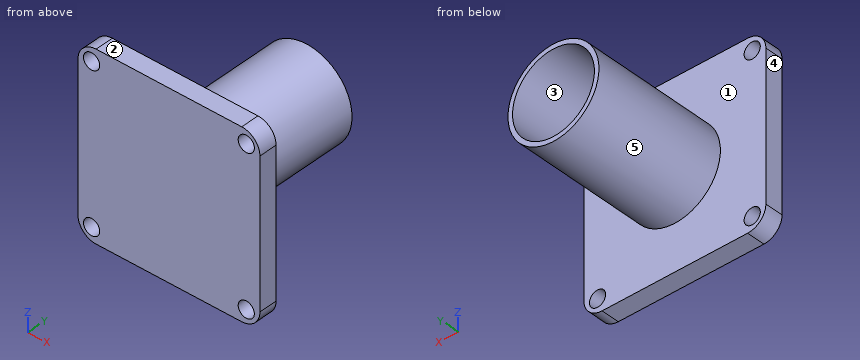
Autodesk Inventor part; units mm, degrees
ref_plane "YZ Plane" through (0, 0, 0) normal (1, 0, 0) x (0, 1, 0)
ref_plane "XZ Plane" through (0, 0, 0) normal (0, 1, 0) x (-1, 0, 0)
sketch "Sketch1" plane through (0, 0, 0) normal (0, 1, 0) x (-1, 0, 0)
  line L0 (-8, 10) -> (8, 10)
  line L1 (10, 8) -> (10, -8)
  line L2 (8, -10) -> (-8, -10)
  line L3 (-10, -8) -> (-10, 8)
  line L4 (-10, 10) -> (10, -10) construction
  line L5 (10, 10) -> (-10, -10) construction
  arc A0 (10, 8) -> (8, 10) centre (8, 8) ccw
  arc A1 (8, -10) -> (10, -8) centre (8, -8) ccw
  arc A2 (-8, 10) -> (-10, 8) centre (-8, 8) ccw
  arc A3 (-10, -8) -> (-8, -10) centre (-8, -8) ccw
  point P0 (0, 0)
  dimension "d0" = 20
  dimension "d1" = 20
  dimension "d34" = 2
  dimension "d35" = 2
  dimension "d36" = 2
  dimension "d37" = 2
extrude "Extrusion1" add sketch "Sketch1" along normal blind 2
sketch "Sketch2" plane through (0, 2, 0) normal (0, 1, 0) x (1, 0, 0)
  line L0 (8.5, -8.5) -> (-8.5, -8.5)
  line L1 (-8.5, -8.5) -> (-8.5, 8.5)
  line L2 (-8.5, 8.5) -> (8.5, 8.5)
  line L3 (8.5, 8.5) -> (8.5, -8.5)
  line L4 (8.5, -8.5) -> (-8.5, 8.5) construction
  line L5 (-8.5, -8.5) -> (8.5, 8.5) construction
  point P0 (0, 0)
  dimension "d4" = 17
  dimension "d5" = 17
hole "Hole1" at (-8.5, 2, 8.5) direction (0, -1, 0) diameter 1.778 end through all
hole "Hole2" at (8.5, 2, 8.5) direction (0, -1, 0) diameter 1.778 end through all
hole "Hole3" at (-8.5, 2, -8.5) direction (0, -1, 0) diameter 1.778 end through all
hole "Hole4" at (8.5, 2, -8.5) direction (0, -1, 0) diameter 1.778 end through all
sketch "Sketch3" plane through (0, 2, 0) normal (0, 1, 0) x (1, 0, 0)
  circle A0 centre (0, 0) radius 5
  dimension "d38" = 10
extrude "Extrusion2" add sketch "Sketch3" along normal blind 15 and the other way blind 1
sketch "Sketch4" plane through (0, 17, 0) normal (0, 1, 0) x (1, 0, 0)
  circle A0 centre (0, 0) radius 4.5
  dimension "d41" = 9
extrude "Extrusion3" cut sketch "Sketch4" against normal blind 15
sketch "Sketch12" plane through (0, 0, 0) normal (0, 0, 1) x (1, 0, 0)
  line L0 (-10, 0) -> (-10, 2) construction
  line L1 (-10, 2) -> (-5, 2) construction
  line L2 (-5, 2) -> (-5, 17) construction
  line L3 (-5, 17) -> (-4.5, 17) construction
  line L4 (-4.5, 17) -> (-4.5, 2) construction
  line L5 (-4.5, 2) -> (4.5, 2) construction
  line L6 (4.5, 2) -> (4.5, 17) construction
  line L7 (4.5, 17) -> (5, 17) construction
  line L8 (5, 17) -> (5, 2) construction
  line L9 (5, 2) -> (10, 2) construction
  line L10 (10, 2) -> (10, 0) construction
  line L11 (10, 0) -> (-10, 0) construction
  line L12 (-5, 17) -> (-8.8394, 7.1494)
  line L13 (-5, 2) -> (5, 2)
  line L14 (-8.8394, 7.1494) -> (-5, 2)
  point P0 (0, 0)
properties part number "mock"
Verification items for the finished model (mm, model axes). Face numbers are marked on the shaded views. A direction names the side the tool comes from. Give positions to 0.01 mm unless a question says otherwise; leave off trailing zeros. Order: outer loops, then holes, each group sorted by start corner. A loop starts at its lowest first (then second) coordinate and runs counter-clockwise, first axis right, second up. Notation, with made-up numbers: M 43,58 L 101,58 A20 ccw 101,76 Z; hole C 55,-15 d1. An arc over 180 degrees is marked long. Answer as a JSON object with one key per item and string values. Group by question number.
1) Access from +Z, -Z, +X, -X, +Y, -Y to the whole of each face (thin tool, end or side, straight path). Record for the marked faces 4 and 5.
2) Cross-section at C-C (y = 13). Enter the section's corners in (x, z), then the cut area to 3 significant figures.
3) Depth check by flat-ended pin: pin 1 Ø3 at (x, z) = (-8.5, -8.5) entering from +Y; pin 2 Ø5 at (x, y) = (-1, 8) entering from -Z; pin 3 Ø6 at (x, y) = (-4, 10.5) entering from +Z. Enter the tip coordinate at first touch or a pass-through.
4) Mould release check, pull along Z, two halves, no side actions. Record for the marked faces 1, 2 and 3: released by +Z, released by -Z, zero draft, split by the parting line, or undercut.
5) Cross-section at D-D (z = 8.5). Enter the section's corners in (x, y).
6) Cross-section at A-A (x = -8.5). Enter the section's corners in (y, z).
7) Scan lines: line 1 along Z through (x, y) = (8.5, 1.45); line 2 along Z through (x, y) = (0, 6.75). Record each from-to range of solid material in increasing order. Write a range as [from, to].
8) Cross-section at B-B (z = 0). Enter the section's corners in (x, y), then the cut area to 3 significant figures.
Result sheet:
{
 "1": {"face 4": "+Z, -Z, -X, +Y, -Y", "face 5": "+Y"},
 "2": {"outline": "C 0,0 d10; hole C 0,0 d9", "area": "14.9 mm2"},
 "3": {"pin 1": "stops at y = 2", "pin 2": "stops at z = -5", "pin 3": "stops at z = 4.9"},
 "4": {"face 1": "zero draft", "face 2": "released by +Z", "face 3": "undercut"},
 "5": {"outline": "M -9.94,0 L -9.39,0 L -9.39,2 L -9.94,2 Z; M -7.61,0 L 7.61,0 L 7.61,2 L -7.61,2 Z; M 9.39,0 L 9.94,0 L 9.94,2 L 9.39,2 Z"},
 "6": {"outline": "M 0,-9.94 L 2,-9.94 L 2,-9.39 L 0,-9.39 Z; M 0,-7.61 L 2,-7.61 L 2,7.61 L 0,7.61 Z; M 0,9.39 L 2,9.39 L 2,9.94 L 0,9.94 Z"},
 "7": {"line 1": "z = [-9.94, -9.39], [-7.61, 7.61], [9.39, 9.94]", "line 2": "z = [-5, -4.5], [4.5, 5]"},
 "8": {"outline": "M -10,0 L 10,0 L 10,2 L 5,2 L 5,17 L 4.5,17 L 4.5,2 L -4.5,2 L -4.5,17 L -5,17 L -5,2 L -10,2 Z", "area": "55.0 mm2"}
}
